Geometry: see drawing. Coordinates: mm, zero at the bounding-box minimum. A direction names the side the tool comes from. Round coordinates to 2 decimals unless told otherwise and drop trailing zeros. Loops run counter-clockwise (first coordinate to the right, second up) from the corner with the lowest first, then second, coordinate; pieces in that order, holes last.
(1) First-contact query: pin 1 Ø7.5 at (x, y) = (106.5, 31) entering from +Z; pin 2 Ø12 at (x, z) = (175.5, 38) entering from -Y; pin 3 Ø7.5 at (x, y) = (100, 27) entering from -Z. Flat tips, straight axial feed; report the tip coordinate or a pass-through.
(2) Cut plane A-A, the plane z = 59. Output: boundary loops of the cut face in (x, y) (3 decimals).
(3) Cut plane C-C, the plane x = 164. Output: boundary loops of the cut face in (y, z) (3 decimals).
(4) Access query for the marked faces 1, 2 and 3. Directions: +Z, -Z, +X, -X, +Y, -Y. A direction counts if a zero-diameter tool reaches every point of the face in a straight line with its end or side. Return the directions, or none.
(5) Line query: line 1 (X direction, y = 53.3, z = 25.4); line 2 (Z direction, x = 25, y = 53); line 3 (Y direction, x = 184, z = 82.5) (3 decimals). Output: solid intervals per line, ascending.
(6) Cut plane B-B, the plane y = 36. Output: boundary loops of the cut face in (x, z), and give its area (3 significant figures).
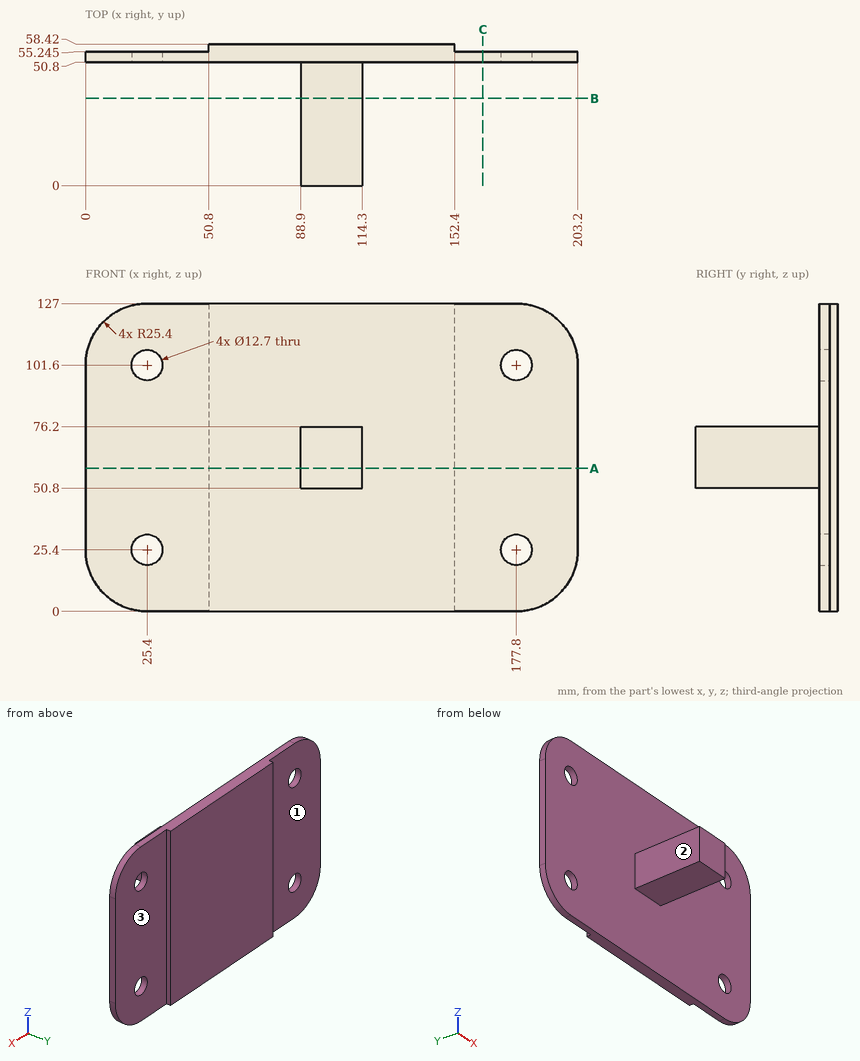
Reported:
1. pin 1: stops at z = 76.2
1. pin 2: stops at y = 50.8
1. pin 3: stops at z = 50.8
2. outline: (0, 50.8) - (88.9, 50.8) - (88.9, 0) - (114.3, 0) - (114.3, 50.8) - (203.2, 50.8) - (203.2, 55.245) - (152.4, 55.245) - (152.4, 58.42) - (50.8, 58.42) - (50.8, 55.245) - (0, 55.245) - close
3. outline: (50.8, 0) - (55.245, 0) - (55.245, 127) - (50.8, 127) - close
4. face 1: +Z, -Z, -X, +Y
4. face 2: +Z, -Z, -X, -Y
4. face 3: +Z, -Z, +X, +Y
5. line 1: x = 0 to 19.05, 31.75 to 171.45, 184.15 to 203.2
5. line 2: z = 0 to 19.06, 31.74 to 95.26, 107.94 to 127
5. line 3: y = 50.8 to 55.245
6. outline: (88.9, 50.8) - (114.3, 50.8) - (114.3, 76.2) - (88.9, 76.2) - close
6. area: 645 mm2
